The model under review builds one solid part; all positions refer to its coordinate system, in mm. Face numbers are marked on the shaded views. Coordinates: 2 decimals unless noted, no trailing zeros.
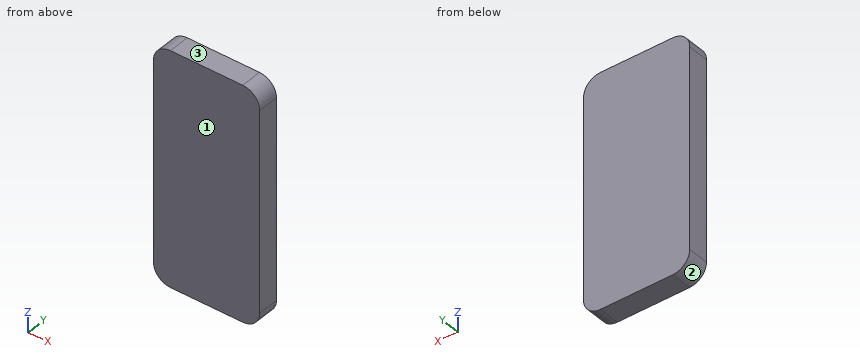
```python
from build123d import *

# Parameters (mm, degrees)
F0_W     = 63.5
F0_H     = 139.7
F1_DEPTH = 12.7
F2_R     = 10.16
F3_R     = 10.16
F4_R     = 10.16
F5_R     = 10.16


with BuildPart() as f1:
    # F0 (on Front) → F1 (new body)
    with BuildSketch(Plane.XZ):
        with Locations((31.75, 69.85)):
            Rectangle(F0_W, F0_H)
    extrude(amount=-F1_DEPTH)

    # F2
    f2_edges = [f1.edges().sort_by_distance(p)[0] for p in [
        (63.5, 6.35, 139.7),
    ]]
    fillet(f2_edges, radius=F2_R)

    # F3
    f3_edges = [f1.edges().sort_by_distance(p)[0] for p in [
        (63.5, 6.35, 0),
    ]]
    fillet(f3_edges, radius=F3_R)

    # F4
    f4_edges = [f1.edges().sort_by_distance(p)[0] for p in [
        (0, 6.35, 139.7),
    ]]
    fillet(f4_edges, radius=F4_R)

    # F5
    f5_edges = [f1.edges().sort_by_distance(p)[0] for p in [
        (0, 6.35, 0),
    ]]
    fillet(f5_edges, radius=F5_R)


solid = f1.part
```
Item 1: For pin 1 (2 mm diameter, centred on x = 56.5, y = 8, fed in from +Z), flat-tipped, find the tip position at first contact; note if it passes through.
Solved:
pin 1: stops at z = 139.47
Item 2: Mouldability with a two-part tool opening along Z and no side actions: class the marked faces 1, 2 and 3 as pulls with the +Z half, pulls with the -Z half, needs draft (parallel to the pull), parting line crosses it, or undercut.
Solved:
face 1: needs draft
face 2: pulls with the -Z half
face 3: pulls with the +Z half
Item 3: To check wall thickness, follow line 1 along Z through (x, y) = (57, 7); line 2 along Z through (x, y) = (5.5, 0.5). State the ranges of each line that lie inside material, in increasing order.
Solved:
line 1: z = 0.68 to 139.02
line 2: z = 1.13 to 138.57
